Part print with two shaded views. Sizes in mm from the minimum x, y, z corner. A direction names the side the tool comes from. Coordinates: 2 decimals unless noted, no trailing zeros. Write each loop counter-clockwise with the first axis right and the second up, starting at its lowest first coordinate (ties: lowest second). Pieces come first, ordered by that corner, then holes. Notation, with made-up numbers: (40.5, 16) - (50.5, 16) arc R24 ccw to (50.5, 52) - close; hole circle Ø8 at (29.25, 61.5). An arc over 180 degrees is marked (long way). One line per question, with ' | ' between items. Start each with the question number.
1. Band-saw the part on A-A, the plane x = 179. Write the cut outline in (y, z), then the cut area to 3 significant figures.
2. Two-plate mould, pull along Y, no slides. Class the marked faces 1, 2 and 3: +Y half, -Y half, draft (parallel to the pull), parting line (faces both ways), or undercut.
3. Probe line 1 (X direction, y = 95.5, z = 53); line 2 (Y direction, x = 269.5, z = 30.5); line 3 (Y direction, x = 197, z = 17.5). List the from-to ranges inside material, lowest first.
4. Band-saw the part on C-C, the plane y = 23.5. Write the cut outline in (x, z), then the cut area to 3 significant figures.
5. Flat gauge pins, fed straight in: P1, Ø8, axis at y = 101.5, z = 87.5, coming from the +X side; P2, Ø17.5, axis at x = 284.5, y = 120, coming from the +Z side; P3, Ø21, axis at x = 155, y = 85, coming from the +Z side. Where does each tip first touch, or does it go through?
6. Band-saw the part on B-B, the plane y = 89. Write the cut outline in (x, z), then the cut area to 3 significant figures.
7. Which spindle directions (+Z, -Z, +X, -X, +Y, -Y) get a long thin tool onto all of the face, cutting with end or side? Do the marked faces 4, 5, 6, 7 and 8. Say none if no direction does.
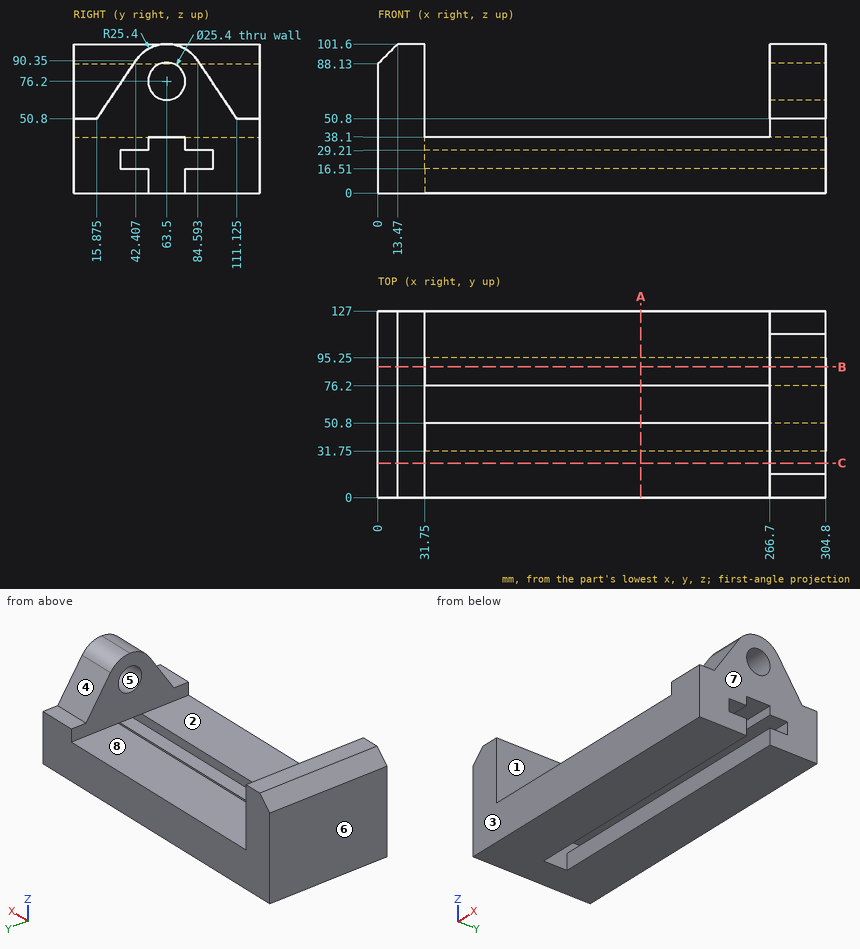
Filled in:
1) outline: (0, 0) - (50.8, 0) - (50.8, 16.51) - (31.75, 16.51) - (31.75, 29.21) - (50.8, 29.21) - (50.8, 38.1) - (0, 38.1) - close; (76.2, 0) - (127, 0) - (127, 38.1) - (76.2, 38.1) - (76.2, 29.21) - (95.25, 29.21) - (95.25, 16.51) - (76.2, 16.51) - close | area: 3,390 mm²
2) face 1: undercut | face 2: draft | face 3: -Y half
3) line 1: x = 0 to 31.75, 266.7 to 304.8 | line 2: y = 0 to 50.8, 76.2 to 127 | line 3: y = 0 to 31.75, 95.25 to 127
4) outline: (0, 0) - (304.8, 0) - (304.8, 62.17) - (266.7, 62.17) - (266.7, 38.1) - (31.75, 38.1) - (31.75, 101.6) - (13.47, 101.6) - (0, 88.13) - close | area: 14,500 mm²
5) P1: stops at x = 31.75 | P2: stops at z = 50.8 | P3: stops at z = 38.1
6) outline: (0, 0) - (304.8, 0) - (304.8, 16.51) - (31.75, 16.51) - (31.75, 29.21) - (304.8, 29.21) - (304.8, 83.78) - (266.7, 83.78) - (266.7, 38.1) - (31.75, 38.1) - (31.75, 101.6) - (13.47, 101.6) - (0, 88.13) - close | area: 11,800 mm²
7) face 4: +Z, +X, +Y | face 5: +X | face 6: +Z, -Z, -X, +Y, -Y | face 7: +Z, -Z, +X, +Y, -Y | face 8: +Z, +Y, -Y
